Verification items for the finished model (mm, model axes). A direction names the side the tool comes from. Coordinates: 2 decimals unless noted, no trailing zeros. Write each loop counter-clockwise with the first axis right and the second up, starting at its lowest first coordinate (ties: lowest second). Pieces come first, ordered by that corner, then holes. Notation, with made-up numbers: (-1, 75.5) -> (47, 75.5) arc R26 ccw to (47, 103.5) -> close; hole circle Ø5 at (65.25, 81). An arc over 180 degrees is marked (long way). Write item = value, one per line. Start each with the question number.
(1) Mould release check, pull along Z, two halves, no side actions. Record for faces 6 (the face through (7.185, -1.437, 1.318)), 7 (the face through (-6, 0, 0)), 8 (the face through (8.76, -0.75, -0.03)): released by +Z, released by -Z, zero draft, split by the parting line, or undercut.
(2) Section check B-B (y = 0). Record the cut outline in (x, z).
(3) Material ranges on probe 1 along Z at (x, y) = (8.8, 0); probe 2 along X at (y, z) = (-1.55, -0.85); probe 3 along X at (y, z) = (-1.4, 0.45), recorded low to high. Write a range as [from, to].
(4) Gauge pin test, flat ends, axial feed: pin 1 Ø1.5 at (y, z) = (1, 0.5) entering from -X; pin 2 Ø1 at (x, y) = (4, 1) entering from +Z; pin 3 Ø1 at (x, y) = (-3.5, 0) entering from -Z; pin 4 Ø1.5 at (x, z) = (-1, 0) entering from +Y. Record the tip position at first contact, or that the pin passes through.
(5) Set-up check for faces 1 (the face through (4.56, -1.27, -0.97)), 2 (the face through (-3, 0, -1.85)), 3 (the face through (-3, 0.45, 0)), 4 (the face through (8.509, 0, 0)), 5 (the face through (-3, -0.45, 0)): record each of +Z, -Z, +X, -X, +Y, -Y from which the full face is reachable in a straight line by a thin tool's end or side.
(6) Section check D-D (z = 1). Record the cut outline in (x, y).
(7) Section check C-C (x = -1.25). Record the cut outline in (y, z), plus the area to 3 significant figures.
(8) Section check A-A (z = 0). Record the cut outline in (x, y), plus the area to 3 significant figures.
Autodesk Inventor part; units mm, degrees
ref_plane "YZ Plane" through (0, 0, 0) normal (1, 0, 0) x (0, 1, 0)
ref_plane "XZ Plane" through (0, 0, 0) normal (0, 1, 0) x (-1, 0, 0)
ref_plane "XY Plane" through (0, 0, 0) normal (0, 0, 1) x (1, 0, 0)
sketch "Sketch1" plane through (0, 0, 0) normal (0, 0, 1) x (1, 0, 0)
  line L0 (0, 0) -> (9.0087, 0)
  line L1 (0, 0) -> (0, 2)
  line L2 (0, 2) -> (3.8, 2)
  line L3 (3.8, 2) -> (3.8, 1.6)
  line L4 (3.8, 1.6) -> (5.3087, 1.6)
  line L5 (5.3087, 1.6) -> (5.3087, 1.95)
  line L6 (5.3087, 1.95) -> (9.0087, 1.95)
  line L7 (9.0087, 1.95) -> (9.0087, 0.75)
  line L8 (9.0087, 0.75) -> (8.5087, 0.75)
  line L9 (8.5087, 0.75) -> (8.5087, 0)
  dimension "d0" = 4
  dimension "d1" = 3.9
  dimension "d2" = 3.8
  dimension "d3" = 3.7
  dimension "d5" = 3.2
  dimension "d10" = 1.5
  dimension "d11" = 0.5
revolve "Revolution1" add sketch "Sketch1" angle 360 about axis through (0, 0, 0) along (1, 0, 0)
sketch "Sketch2" plane through (0, 0, 0) normal (-1, 0, 0) x (0, 0, 1)
  line L0 (-1.85, -0.45) -> (1.85, -0.45)
  line L1 (1.85, -0.45) -> (1.85, 0.45)
  line L2 (1.85, 0.45) -> (-1.85, 0.45)
  line L3 (-1.85, 0.45) -> (-1.85, -0.45)
  line L4 (-1.85, -0.45) -> (1.85, 0.45) construction
  line L5 (1.85, -0.45) -> (-1.85, 0.45) construction
  point P0 (0, 0)
  dimension "d6" = 3.7
  dimension "d7" = 0.9
extrude "Extrusion1" add sketch "Sketch2" along normal blind 6
properties part number "laser_realpoo_4mm" material "Brass, Soft Yellow"
Response:
q1.face_6 = split by the parting line
q1.face_7 = zero draft
q1.face_8 = undercut
q2.outline = (-6, -1.85) -> (0, -1.85) -> (0, -2) -> (3.8, -2) -> (3.8, -1.6) -> (5.31, -1.6) -> (5.31, -1.95) -> (9.01, -1.95) -> (9.01, -0.75) -> (8.51, -0.75) -> (8.51, 0.75) -> (9.01, 0.75) -> (9.01, 1.95) -> (5.31, 1.95) -> (5.31, 1.6) -> (3.8, 1.6) -> (3.8, 2) -> (0, 2) -> (0, 1.85) -> (-6, 1.85) -> close
q3.probe_1 = [-1.95, -0.75], [0.75, 1.95]
q3.probe_2 = [0, 3.8], [5.31, 9.01]
q3.probe_3 = [0, 9.01]
q4.pin_1 = -6
q4.pin_2 = 1.93
q4.pin_3 = -1.85
q4.pin_4 = 0.45
q5.face_1 = none
q5.face_2 = -Z, -X, +Y, -Y
q5.face_3 = +Z, -Z, -X, +Y
q5.face_4 = +X
q5.face_5 = +Z, -Z, -X, -Y
q6.outline = (-6, -0.45) -> (0, -0.45) -> (0, -1.73) -> (3.8, -1.73) -> (3.8, -1.25) -> (5.31, -1.25) -> (5.31, -1.67) -> (9.01, -1.67) -> (9.01, 1.67) -> (5.31, 1.67) -> (5.31, 1.25) -> (3.8, 1.25) -> (3.8, 1.73) -> (0, 1.73) -> (0, 0.45) -> (-6, 0.45) -> close
q7.outline = (-0.45, -1.85) -> (0.45, -1.85) -> (0.45, 1.85) -> (-0.45, 1.85) -> close
q7.area = 3.33 mm2
q8.outline = (-6, -0.45) -> (0, -0.45) -> (0, -2) -> (3.8, -2) -> (3.8, -1.6) -> (5.31, -1.6) -> (5.31, -1.95) -> (9.01, -1.95) -> (9.01, -0.75) -> (8.51, -0.75) -> (8.51, 0.75) -> (9.01, 0.75) -> (9.01, 1.95) -> (5.31, 1.95) -> (5.31, 1.6) -> (3.8, 1.6) -> (3.8, 2) -> (0, 2) -> (0, 0.45) -> (-6, 0.45) -> close
q8.area = 39.1 mm2
